The figure shows three views and two pictorial views of one solid part (mm, origin at its lowest corner). Answer the questions. A direction names the side the tool comes from. Give positions to 0.01 mm unless a question says otherwise; leave off trailing zeros. Order: outer loops, then holes, each group sorted by start corner. A loop starts at its lowest first (then second) coordinate and runs counter-clockwise, first axis right, second up. Notation, with made-up numbers: (-35.5, 35.25) - (11.5, 35.25) arc R11 ccw to (11.5, 56.25) - close; hole circle Ø8 at (-11, 7.25). An arc over 180 degrees is marked (long way). Return JSON: item names as keys, results as strings. Group by question number.
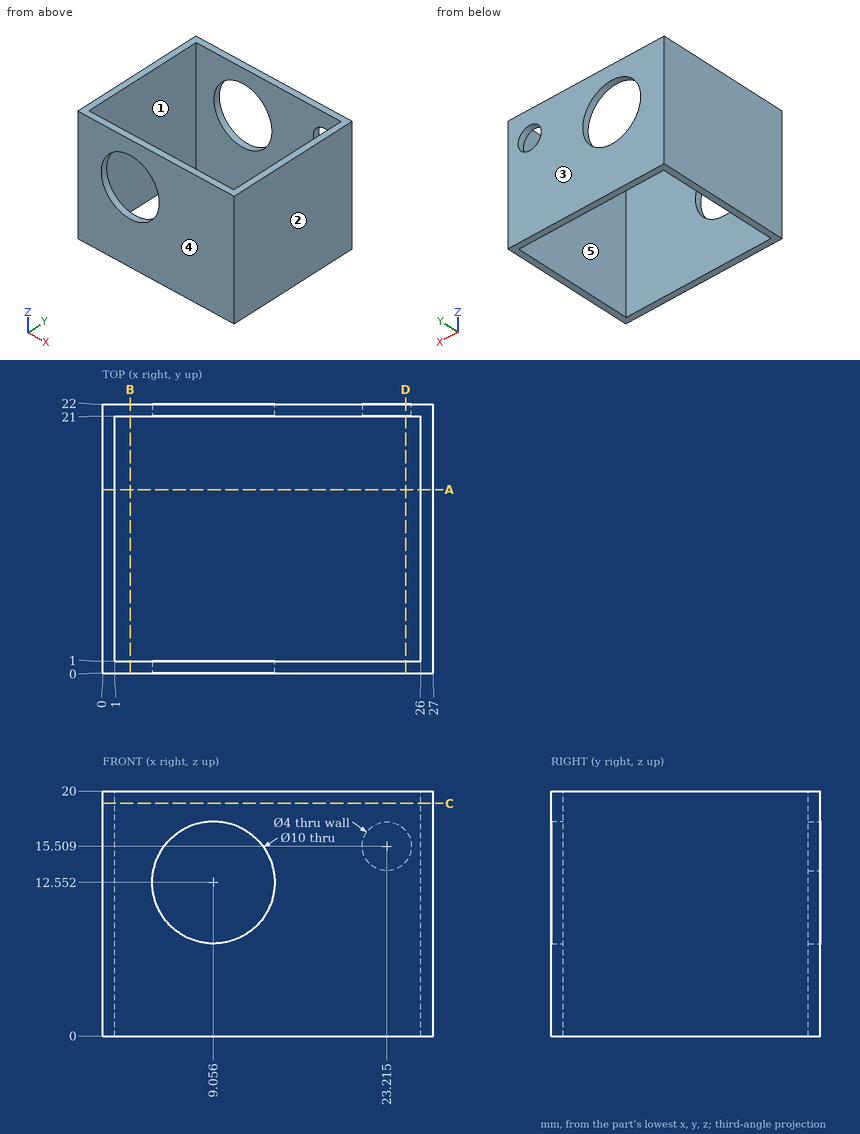
1. Determine the mould class of the marked faces 1, 2 and 3 for opening direction Y: released by +Y, released by -Y, zero draft, split by the parting line, or undercut.
2. This flat-tipped pin is pushed along its axis until it touches: pin 1 (8 mm diameter, centred on x = 9.06, z = 12.55, fed in from -Y). Where does it stop, or does it pass through?
3. The part is cut by section D-D (x = 24.75). Give the vertices of the cut face in (y, z).
4. The part is cut by section B-B (x = 2.25). Give the vertices of the cut face in (y, z).
5. The part is cut by section C-C (z = 19). Give the vertices of the cut face in (x, y).
6. A tool of negligible diameter and unlimited length cuts with its end or side. For the marked faces 4 and 5, from which of +Z, -Z, +X, -X, +Y, -Y can it reach the whole face along a straight path? Write none if from no direction.
7. The part is cut by section A-A (y = 15). Give the vertices of the cut face in (x, z).
8. Consider probe 1 along Y at (x, z) = (22.75, 11.25); probe 2 along X at (y, z) = (12.75, 16.75). Determine where each line is inside the solid, lowest interval first. Write a range as from..to.
Answers:
{
 "1": {"face 1": "undercut", "face 2": "zero draft", "face 3": "released by +Y"},
 "2": {"pin 1": "passes through"},
 "3": {"outline": "(0, 0) - (1, 0) - (1, 20) - (0, 20) - close; (21, 0) - (22, 0) - (22, 14.23) - (21, 14.23) - close; (21, 16.79) - (22, 16.79) - (22, 20) - (21, 20) - close"},
 "4": {"outline": "(0, 0) - (1, 0) - (1, 20) - (0, 20) - close; (21, 0) - (22, 0) - (22, 20) - (21, 20) - close"},
 "5": {"outline": "(0, 0) - (27, 0) - (27, 22) - (0, 22) - close; hole (1, 1) - (26, 1) - (26, 21) - (1, 21) - close"},
 "6": {"face 4": "+Z, -Z, +X, -X, -Y", "face 5": "+Z, -Z"},
 "7": {"outline": "(0, 0) - (1, 0) - (1, 20) - (0, 20) - close; (26, 0) - (27, 0) - (27, 20) - (26, 20) - close"},
 "8": {"probe 1": "y = 0..1, 21..22", "probe 2": "x = 0..1, 26..27"}
}
